```python
from build123d import *

# Parameters (mm, degrees)
F1_DEPTH = 20
F2_W     = 20
F2_H     = 60
F3_DEPTH = 30


with BuildPart() as f1:
    # F0 (on Front) → F1 (new body)
    with BuildSketch(Plane.XZ):
        Polygon((-40, 30), (-40, -30), (40, -30), (40, 0), (10, 30), align=None)
    extrude(amount=F1_DEPTH)

    # F2 (on face) → F3 (join)
    with BuildSketch(Plane.XZ.offset(20)):
        with Locations((-30, 0)):
            Rectangle(F2_W, F2_H)
    extrude(amount=F3_DEPTH)


solid = f1.part
```
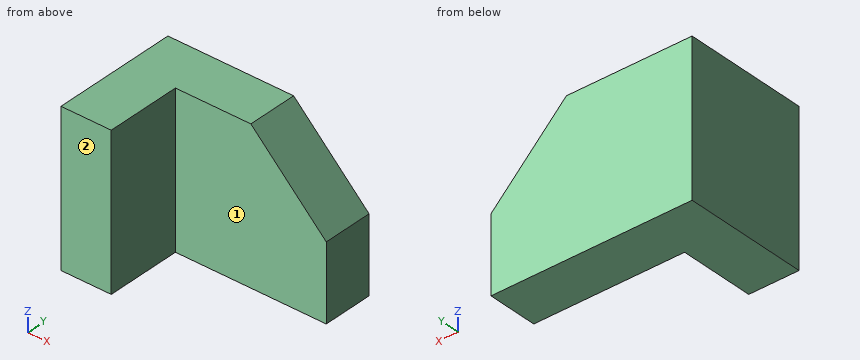
Verification items for the finished model (mm, model axes). Face numbers are marked on the shaded views. A direction names the side the tool comes from. Give positions to 0.01 mm unless a question says otherwise; leave off trailing zeros. Order: outer loops, then holes, each group sorted by start corner. A loop starts at its lowest first (then second) coordinate and runs counter-clockwise, first axis right, second up. Notation, with made-up numbers: (88, 56.5) -> (134, 56.5) arc R17 cw to (134, 65.5) -> close; hole circle Ø11 at (60.5, 22). An arc over 180 degrees is marked (long way). Use a Markdown table: item, result.
1) Material ranges on probe 1 along X at (y, z) = (-24.5, 4); probe 2 along Y at (x, z) = (-5, -6); probe 3 along X at (y, z) = (-2.5, 18.5), recorded low to high.
Results:
| item | result |
|---|---|
| probe 1 | -40 to -20 |
| probe 2 | -20 to 0 |
| probe 3 | -40 to 21.5 |
2) Section check C-C, the plane x = 13.5. Record the boundary of the cut face in (y, z), then the cut area to 3 significant figures.
Results:
| item | result |
|---|---|
| outline | (-20, -30) -> (0, -30) -> (0, 26.5) -> (-20, 26.5) -> close |
| area | 1,130 mm² |
3) Section check A-A, the plane y = -8. Record the boundary of the cut face in (x, z), then the cut area to 3 significant figures.
Results:
| item | result |
|---|---|
| outline | (-40, -30) -> (40, -30) -> (40, 0) -> (10, 30) -> (-40, 30) -> close |
| area | 4,350 mm² |
4) Section check D-D, the plane z = -14. Record the boundary of the cut face in (x, y), then the cut area to 3 significant figures.
Results:
| item | result |
|---|---|
| outline | (-40, -50) -> (-20, -50) -> (-20, -20) -> (40, -20) -> (40, 0) -> (-40, 0) -> close |
| area | 2,200 mm² |
5) Depth check by flat-ended pin: pin 1 Ø1 at (y, z) = (-28, 15) entering from +X; pin 2 Ø1.5 at (x, y) = (-18, -22) entering from -Z; pin 3 Ø1 at (x, y) = (28.5, -20) entering from +Z; pin 4 Ø3 at (x, z) = (-4, -10.5) entering from -Y. Enter the tip coordinate at first touch or a pass-through.
Results:
| item | result |
|---|---|
| pin 1 | x = -20 |
| pin 2 | through |
| pin 3 | z = 12 |
| pin 4 | y = -20 |
6) Tool access check on the marked faces 1 and 2. Record the directions out of +Z, -Z, +X, -X, +Y, -Y that give a thin tool (end or side, any length) a straight path to the whole face; none if there is none.
Results:
| item | result |
|---|---|
| face 1 | +Z, -Z, +X, -Y |
| face 2 | +Z, -Z, +X, -X, -Y |
7) Section check B-B, the plane z = 19. Record the boundary of the cut face in (x, y).
Results:
| item | result |
|---|---|
| outline | (-40, -50) -> (-20, -50) -> (-20, -20) -> (21, -20) -> (21, 0) -> (-40, 0) -> close |
